Input: dimensioned drawing with shaded views. Units: mm. Origin: part minimum x, y, z. Give positions to 0.01 mm unless a question says otherwise; leave off trailing zeros. Write each loop counter-clockwise with the first axis right and the second up, starting at its lowest first coordinate (ties: lowest second). Pieces come first, ordered by that corner, then holes. Notation, with made-up numbers: (-33, 68) - (23, 68) arc R21 cw to (23, 83) - close; hole circle Ø11 at (-31.5, 68). An arc over 180 degrees is marked (long way). Answer as CSV lines item,"result".
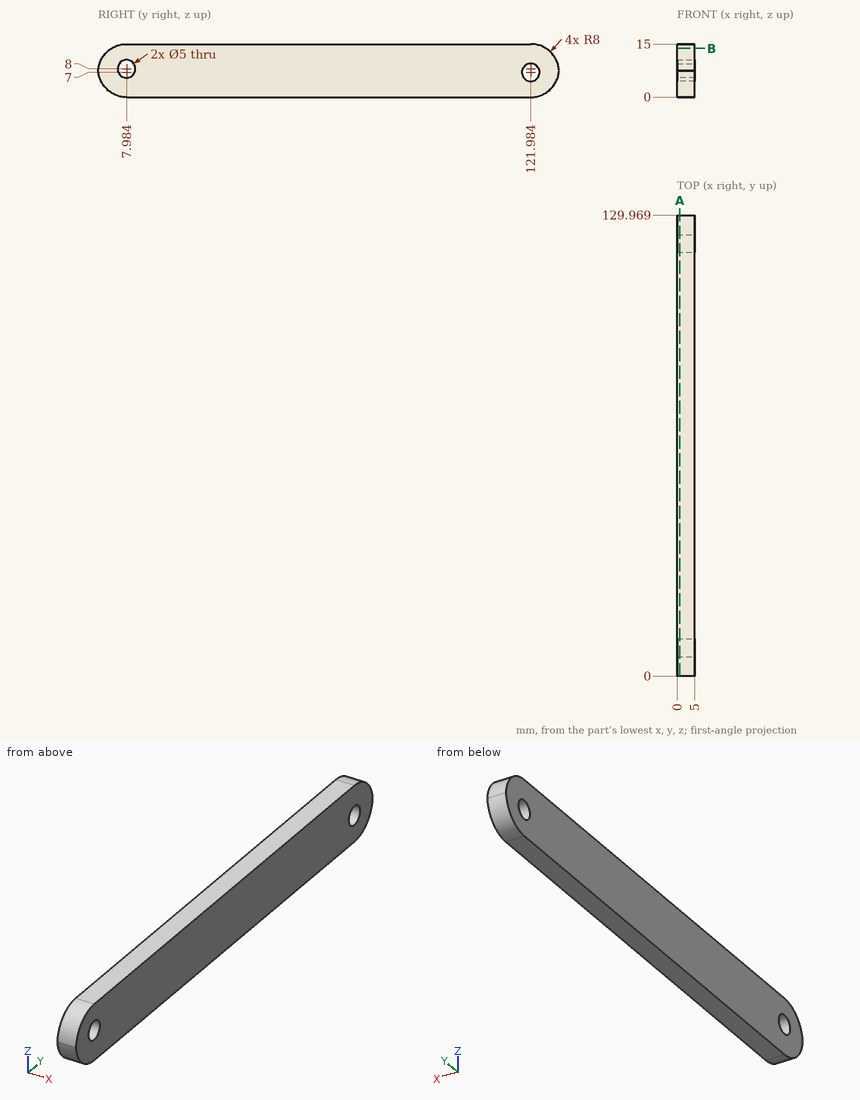
Item 1: Cut plane A-A on x = 0.8. Return the cut outline in (y, z) (1 decimal).
The answers:
outline,"(0, 7.5) arc R8 ccw to (8, 0) - (122, 0) arc R8 ccw to (130, 7.5) arc R8 ccw to (122, 15) - (8, 15) arc R8 ccw to start; hole circle Ø5 at (8, 8); hole circle Ø5 at (122, 7)"
Item 2: Ray query, line 1 (Y direction, x = 2.9, z = 7) (1 decimal); line 2 (Y direction, x = 3.45, z = 8) (1 decimal); line 3 (Y direction, x = 2.2, z = 5) (1 decimal). Return the intervals inside material, ascending. Write a range as from..to.
The answers:
line 1,"0..5.7, 10.3..119.5, 124.5..129.9"
line 2,"0..5.5, 10.5..119.7, 124.3..129.9"
line 3,"0.6..120.5, 123.5..129.4"
Item 3: Cut plane B-B on z = 13.75. Return the cut outline in (x, y).
The answers:
outline,"(0, 3.69) - (5, 3.69) - (5, 126.28) - (0, 126.28) - close"
